Verification items for the finished model (mm, model axes). Face numbers are marked on the shaded views. A direction names the side the tool comes from. Coordinates: 2 decimals unless noted, no trailing zeros. Write each loop counter-clockwise with the first axis right and the second up, starting at its lowest first coordinate (ties: lowest second). Pieces come first, ordered by that corner, then holes. Notation, with made-up numbers: (21.25, 25.25) -> (47.25, 25.25) arc R14 ccw to (47.25, 41.25) -> close; hole circle Ø2 at (77, 23.25). An arc over 180 degrees is marked (long way). Answer in a Markdown table with one row per item.
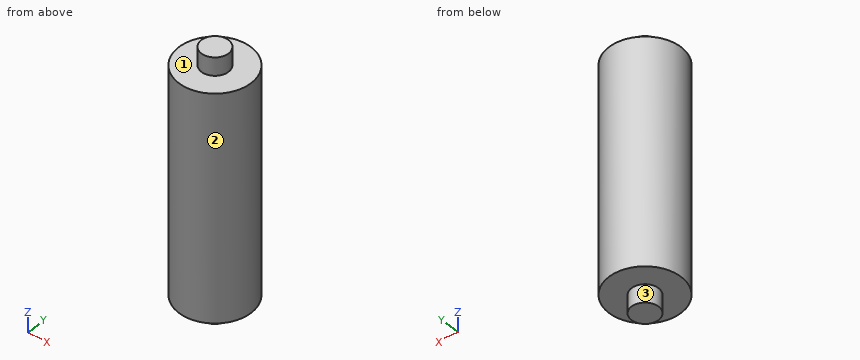
```python
from build123d import *

# Parameters (mm, degrees)
SKETCH1_R           = 40
BOSS_EXTRUDE1_DEPTH = 250
SKETCH2_R           = 15
BOSS_EXTRUDE2_DEPTH = 20


with BuildPart() as part:
    # Sketch1 → Boss-Extrude1 (new body)
    with BuildSketch(Plane.XY):
        Circle(SKETCH1_R)
    extrude(amount=BOSS_EXTRUDE1_DEPTH)

    # Sketch2 → Boss-Extrude2 (add)
    with BuildSketch(Plane.XY.offset(250)):
        Circle(SKETCH2_R)
    boss_extrude2 = extrude(amount=BOSS_EXTRUDE2_DEPTH)

    # Mirror1: Boss-Extrude2 across plane
    add(boss_extrude2.mirror(Plane.XY.offset(125)))


solid = part.part
```
1. Thickness scan on line 1 (Z direction, x = -17, y = -26); line 2 (Y direction, x = -1, z = 251); line 3 (X direction, y = -1, z = 209). Record the ranges inside material, lowest first. Write a range as from..to.
Geometry says:
| item | result |
|---|---|
| line 1 | 0..250 |
| line 2 | -14.97..14.97 |
| line 3 | -39.99..39.99 |
2. Tool access check on the marked faces 1, 2 and 3. Record the directions out of +Z, -Z, +X, -X, +Y, -Y that give a thin tool (end or side, any length) a straight path to the whole face; none if there is none.
Geometry says:
| item | result |
|---|---|
| face 1 | +Z |
| face 2 | +Z, -Z |
| face 3 | -Z |
3. Section check C-C, the plane z = 151.5. Record the boundary of the cut face in (x, y).
Geometry says:
| item | result |
|---|---|
| outline | circle Ø80 at (0, 0) |
4. Depth check by flat-ended pin: P1, Ø8, axis at x = 25, y = -11, coming from the -Z side; P2, Ø4, axis at x = 18.5, y = -21.5, coming from the +Z side; P3, Ø8, axis at x = 8, z = 202, coming from the -Y side. Enter the tip coordinate at first touch or a pass-through.
Geometry says:
| item | result |
|---|---|
| P1 | z = 0 |
| P2 | z = 250 |
| P3 | y = -39.8 |
5. Section check A-A, the plane y = 0. Record the boundary of the cut face in (x, z), plus the area to 3 significant figures.
Geometry says:
| item | result |
|---|---|
| outline | (-40, 0) -> (-15, 0) -> (-15, -20) -> (15, -20) -> (15, 0) -> (40, 0) -> (40, 250) -> (15, 250) -> (15, 270) -> (-15, 270) -> (-15, 250) -> (-40, 250) -> close |
| area | 21,200 mm^2 |
6. Section check D-D, the plane x = 25. Record the boundary of the cut face in (y, z), plus the area to 3 significant figures.
Geometry says:
| item | result |
|---|---|
| outline | (-31.22, 0) -> (31.22, 0) -> (31.22, 250) -> (-31.22, 250) -> close |
| area | 15,600 mm^2 |
